For this review, take the finished solid that the model builds, in its own axes (mm). Round coordinates to 2 decimals unless told otherwise and drop trailing zeros. Write each loop counter-clockwise with the first axis right and the second up, starting at its lowest first coordinate (ties: lowest second). Pieces come first, ordered by that corner, then holes. Notation, with made-up numbers: M 20.25,27.5 L 73.25,27.5 A18 cw 73.25,62.5 Z; hole C 68.5,44 d3. An arc over 180 degrees is marked long. Answer in a Markdown table with one row per item.
```python
from build123d import *

# Parameters (mm, degrees)
SKETCH1_R           = 2.4
BOSS_EXTRUDE1_DEPTH = 6


with BuildPart() as part:
    # Sketch1 → Boss-Extrude1 (new body)
    with BuildSketch(Plane(origin=(0, 0, 0), x_dir=(1, 0, 0), z_dir=(0, 1, 0))):
        with BuildLine():
            ThreePointArc((-35, -32), (-34.121320344, -34.121320344), (-32, -35))
            Line((-32, -35), (94.221825407, -35))
            ThreePointArc((94.221825407, -35), (96.993464004, -33.148050297), (96.343145751, -29.878679656))
            Line((96.343145751, -29.878679656), (-29.878679656, 96.343145751))
            ThreePointArc((-29.878679656, 96.343145751), (-33.148050297, 96.993464004), (-35, 94.221825407))
            Line((-35, 94.221825407), (-35, -32))
        make_face()
        with Locations((-22.980970389, -22.980970389)):
            Circle(SKETCH1_R, mode=Mode.SUBTRACT)
        with Locations((22.980970389, -22.980970389)):
            Circle(SKETCH1_R, mode=Mode.SUBTRACT)
        with Locations((-22.980970389, 22.980970389)):
            Circle(SKETCH1_R, mode=Mode.SUBTRACT)
        with Locations((22.980970389, 22.980970389)):
            Circle(SKETCH1_R, mode=Mode.SUBTRACT)
    extrude(amount=BOSS_EXTRUDE1_DEPTH)


solid = part.part
```
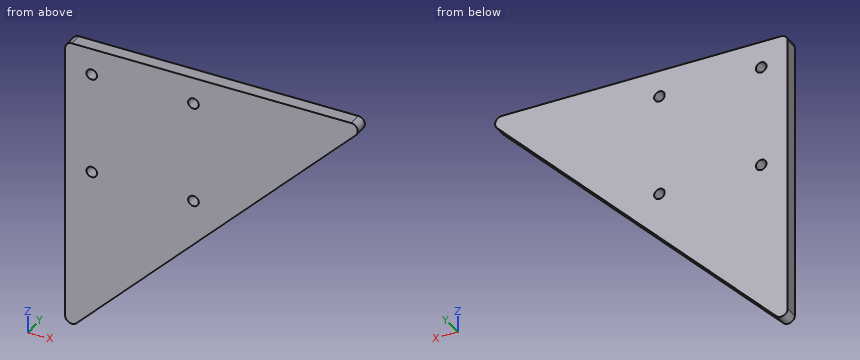
Q1. Insertion check: P1, Ø1.5, axis at y = 3, z = -66, coming from the +X side. The pin has a flat end and moves straight along its axis. Give the tip position at first contact, or say it passes through.
Found:
| item | result |
|---|---|
| P1 | x = 1.21 |
Q2. For probe 1 along X at (y, z) = (5.25, 18.5); probe 2 along X at (y, z) = (2.05, 9); probe 3 along Z at (x, y) = (58.5, 0.8), list the stretches that pass through material, from the lowest coordinate up.
Found:
| item | result |
|---|---|
| probe 1 | -35 to 84.96 |
| probe 2 | -35 to 75.46 |
| probe 3 | -7.96 to 35 |
Q3. Take a section at C-C (z = 15.5). State the section outline as (x, y) points, then the cut area to 3 significant figures.
Found:
| item | result |
|---|---|
| outline | M -35,0 L 81.96,0 L 81.96,6 L -35,6 Z |
| area | 702 mm² |
Q4. Take a section at B-B (x = 72). State the section outline as (y, z) points, then the cut area to 3 significant figures.
Found:
| item | result |
|---|---|
| outline | M 0,5.54 L 6,5.54 L 6,35 L 0,35 Z |
| area | 177 mm² |
Q5. Take a section at A-A (y = 3.6). State the section outline as (x, z) points, then the cut area to 3 significant figures.
Found:
| item | result |
|---|---|
| outline | M -35,-94.22 A3 ccw -29.88,-96.34 L 96.34,29.88 A3 ccw 94.22,35 L -32,35 A3 ccw -35,32 Z; hole C -22.98,-22.98 d4.8; hole C -22.98,22.98 d4.8; hole C 22.98,-22.98 d4.8; hole C 22.98,22.98 d4.8 |
| area | 9,210 mm² |
